```python
from build123d import *

# Parameters (mm, degrees)
SKETCH_R  = 1.1
PAD_DEPTH = 2


with BuildPart() as part:
    # Sketch → Pad (new body)
    with BuildSketch(Plane.XY):
        with BuildLine():
            ThreePointArc((-124.238101, 46.063372), (-127.232991, 44.790439), (-128.810202, 41.944014))
            Line((-128.810202, 41.944014), (-139.403415, -18.133082))
            ThreePointArc((-139.403415, -18.133082), (-138.575137, -21.869205), (-135.347617, -23.925361))
            Line((-135.347617, -23.925361), (-92.569259, -31.46834))
            ThreePointArc((-88.4375, -36.392379), (-89.607278, -33.178441), (-92.569259, -31.46834))
            Line((-88.4375, -36.392379), (-88.4375, -47.34526))
            ThreePointArc((-88.4375, -47.34526), (-87.267722, -50.559198), (-84.305741, -52.269298))
            Line((-84.305741, -52.269298), (-33.428165, -61.240388))
            ThreePointArc((-33.428165, -61.240388), (-29.103544, -61.809735), (-24.745757, -62))
            Line((-24.745757, -62), (24.745757, -62))
            ThreePointArc((24.745757, -62), (29.103544, -61.809735), (33.428165, -61.240388))
            Line((84.305741, -52.269298), (33.428165, -61.240388))
            ThreePointArc((84.305741, -52.269298), (87.267722, -50.559198), (88.4375, -47.34526))
            Line((88.4375, -36.392379), (88.4375, -47.34526))
            ThreePointArc((92.569259, -31.46834), (89.607278, -33.178441), (88.4375, -36.392379))
            Line((135.347617, -23.925361), (92.569259, -31.46834))
            ThreePointArc((135.347617, -23.925361), (138.575137, -21.869205), (139.403415, -18.133082))
            Line((128.810202, 41.944014), (139.403415, -18.133082))
            ThreePointArc((128.810202, 41.944014), (127.232991, 44.790439), (124.238101, 46.063372))
            Line((124.238101, 46.063372), (64.358799, 50.288605))
            ThreePointArc((64.358799, 50.288605), (52.157015, 49.653007), (40.473702, 46.077018))
            Line((40.473702, 46.077018), (15.926856, 35.129447))
            ThreePointArc((15.926856, 35.129447), (11.611572, 31.440305), (10, 25.996567))
            Line((10, 3), (10, 25.996567))
            ThreePointArc((7, 0), (9.12132, 0.87868), (10, 3))
            Line((-7, 0), (7, 0))
            ThreePointArc((-10, 3), (-9.12132, 0.87868), (-7, 0))
            Line((-10, 3), (-10, 25.996567))
            ThreePointArc((-10, 25.996567), (-11.611572, 31.440305), (-15.926856, 35.129447))
            Line((-40.473702, 46.077018), (-15.926856, 35.129447))
            ThreePointArc((-40.473702, 46.077018), (-52.157015, 49.653007), (-64.358799, 50.288605))
            Line((-124.238101, 46.063372), (-64.358799, 50.288605))
        make_face()
        with Locations((123.886163, 41.075773)):
            Circle(SKETCH_R, mode=Mode.SUBTRACT)
        with Locations((134.479376, -19.001323)):
            Circle(SKETCH_R, mode=Mode.SUBTRACT)
        with Locations((83.4375, -47.34526)):
            Circle(SKETCH_R, mode=Mode.SUBTRACT)
        with Locations((20, -57)):
            Circle(SKETCH_R, mode=Mode.SUBTRACT)
        with Locations((-20, -57)):
            Circle(SKETCH_R, mode=Mode.SUBTRACT)
        with Locations((-83.4375, -47.34526)):
            Circle(SKETCH_R, mode=Mode.SUBTRACT)
        with Locations((-134.479376, -19.001323)):
            Circle(SKETCH_R, mode=Mode.SUBTRACT)
        with Locations((-64.77, 41.995)):
            Circle(SKETCH_R, mode=Mode.SUBTRACT)
        with Locations((-123.886163, 41.075773)):
            Circle(SKETCH_R, mode=Mode.SUBTRACT)
        with Locations((64.77, 41.995)):
            Circle(SKETCH_R, mode=Mode.SUBTRACT)
    extrude(amount=PAD_DEPTH)


solid = part.part
```
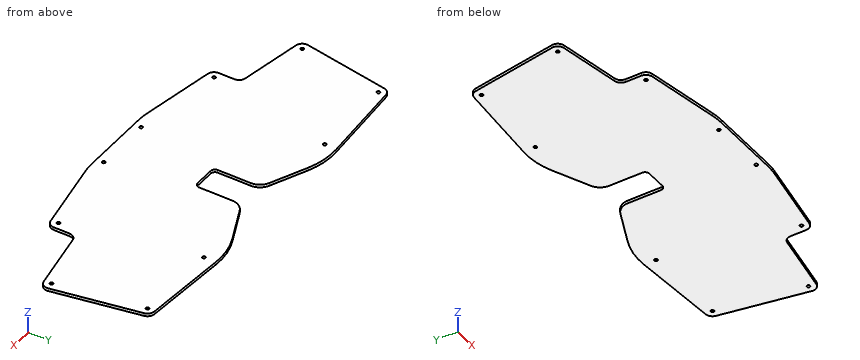
Geometry: final body of the model. Coordinates: model frame, mm. Coordinates: 2 decimals unless noted, no trailing zeros. Order: outer loops, then holes, each group sorted by start corner. A loop starts at its lowest first (then second) coordinate and runs counter-clockwise, first axis right, second up. Notation, with made-up numbers: (72.25, -17.5) - (116.25, -17.5) arc R9 ccw to (116.25, -6.5) - close; hole circle Ø8 at (87, 40.5). An arc over 180 degrees is marked (long way). Return JSON: item names as keys, results as strings. Group by question number.
1. Material intervals for line 1 along X through (y, z) = (-42.5, 0.25); line 2 along X through (y, z) = (15, 1.85); line 3 along X through (y, z) = (-36, 0.95), sorted ascending. Write a range as [from, to].
2. Pin query (flat end, axial travel): pin 1 (1 mm diameter, centred on x = 37, z = 1.5, fed in from -Y). Return the tip coordinate at first contact, or that it passes through.
3. Cut plane C-C (z = 0.8). Count the separate pieces of the cut face and the enclosed holes in it, plus the area to 3 significant figures.
4. Cut plane B-B (y = -26.5). Output: boundary loops of the cut face in (x, z).
5. Cut plane A-A (x = -30). Output: boundary loops of the cut face in (y, z).
Resolved:
{
 "1": {"line 1": "x = [-88.44, 88.44]", "line 2": "x = [-133.56, -10], [10, 133.56]", "line 3": "x = [-88.45, 88.45]"},
 "2": {"pin 1": "stops at y = -60.7"},
 "3": {"separate pieces": "1", "enclosed holes": "10", "area": "24,300 mm²"},
 "4": {"outline": "(-120.75, 0) - (120.75, 0) - (120.75, 2) - (-120.75, 2) - close"},
 "5": {"outline": "(-61.72, 0) - (41.41, 0) - (41.41, 2) - (-61.72, 2) - close"}
}
